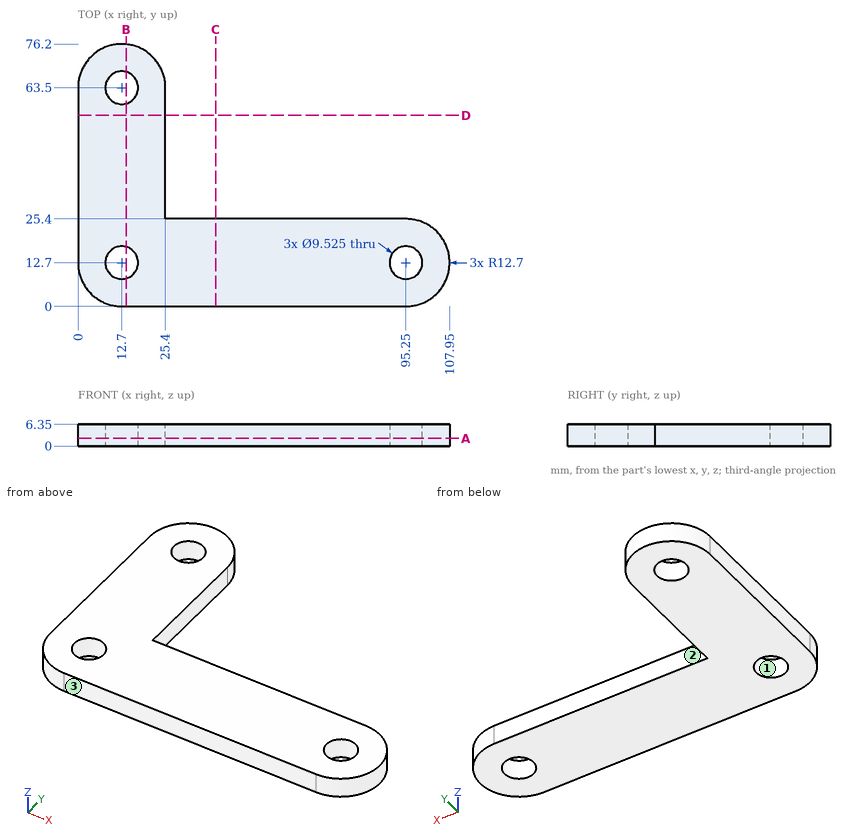
For this review, use the dimensioned drawing (mm, ordinates from the lowest corner) and the shaded views. Coordinates: 2 decimals unless noted, no trailing zeros. Loops run counter-clockwise (first coordinate to the right, second up) from the corner with the lowest first, then second, coordinate; pieces in that order, holes last. Notation, with made-up numbers: (0, -8.75) - (17, -8.75) arc R21 cw to (17, 3.25) - close; hole circle Ø3 at (29, 85.25). An arc over 180 degrees is marked (long way). Use CSV: the item, a comma, the result in double quotes. Start each with the question number.
1) Consider section A-A on z = 2.25. Give the number of separate pieces and of enclosed holes in the cut face, then the cut area to 3 significant figures.
2) Consider section B-B on x = 14. Write out the cut boundary in (y, z).
3) The part is to be moulded in two halves that separate along Y. For the marked faces 1, 2 and 3, say which applies: +Y half, -Y half, draft (parallel to the pull), parting line (faces both ways), or undercut.
4) Wall thickness on L1, parallel to Y at x = 54.5, z = 1; L2, parallel to Y at x = 95.25, z = 1.5; L3, parallel to Y at x = 91, z = 1.25: over which ranges is each line inside the solid? List them lowest first. Write a range as from..to.
5) For pin 1 Ø1.9 at (y, z) = (50.5, 2.5) entering from +X; pin 2 Ø3 at (x, z) = (53, 2.5) entering from +Y; pin 3 Ø2 at (y, z) = (19, 4.5) entering from +X, all flat-tipped, find the tip position at first contact; note any pin that passes through.
6) Consider section C-C on x = 40. Write out the cut boundary in (y, z).
Geometry says:
1,separate pieces,"1"
1,enclosed holes,"3"
1,area,"3,650 mm^2"
2,outline,"(0, 0) - (8.12, 0) - (8.12, 6.35) - (0, 6.35) - close; (17.28, 0) - (58.92, 0) - (58.92, 6.35) - (17.28, 6.35) - close; (68.08, 0) - (76.13, 0) - (76.13, 6.35) - (68.08, 6.35) - close"
3,face 1,"undercut"
3,face 2,"+Y half"
3,face 3,"-Y half"
4,L1,"0..25.4"
4,L2,"0..7.94, 17.46..25.4"
4,L3,"0..10.55, 14.85..25.4"
5,pin 1,"x = 25.4"
5,pin 2,"y = 25.4"
5,pin 3,"x = 106.79"
6,outline,"(0, 0) - (25.4, 0) - (25.4, 6.35) - (0, 6.35) - close"
